Input: part model. Units: mm. Frame: model coordinates. Coordinates: 2 decimals unless noted, no trailing zeros. Write each loop counter-clockwise with the first axis right and the second up, starting at its lowest first coordinate (ties: lowest second). Pieces come first, ordered by that corner, then holes. Notation, with made-up numbers: M 71.5,28.25 L 95.5,28.25 A14 cw 95.5,55.25 Z; hole C 87,43.25 d8. An arc over 180 degrees is marked long. Use one line per item in the form item = value.
from build123d import *

# Parameters (mm, degrees)
SKETCH_1_W          = 207
SKETCH_1_H          = 75
EXTRUDE_1_DEPTH     = 1
SKETCH_2_R          = 3.3
CUT_EXTRUDE_1_DEPTH = 111.088600681
FILLET_1_R          = 5


with BuildPart() as part:
    # 草图1 → 凸台-拉伸1 (new body)
    with BuildSketch(Plane.XY):
        Rectangle(SKETCH_1_W, SKETCH_1_H)
    extrude(amount=EXTRUDE_1_DEPTH)

    # 草图2 → 切除-拉伸1 (cut, through all)
    with BuildSketch(Plane.XY.offset(1)):
        with Locations((-78.5, 29.5)):
            Circle(SKETCH_2_R)
        with Locations((78.5, 29.5)):
            Circle(SKETCH_2_R)
        with Locations((-78.5, -29.5)):
            Circle(SKETCH_2_R)
        with Locations((78.5, -29.5)):
            Circle(SKETCH_2_R)
    extrude(amount=-CUT_EXTRUDE_1_DEPTH, mode=Mode.SUBTRACT)

    # 圆角1
    fillet_1_edges = [part.edges().sort_by_distance(p)[0] for p in [
        (103.5, -37.5, 0.5),
        (-103.5, -37.5, 0.5),
        (-103.5, 37.5, 0.5),
        (103.5, 37.5, 0.5),
    ]]
    fillet(fillet_1_edges, radius=FILLET_1_R)


solid = part.part
(1) Pull-direction query (X, two-part tool) for faces 1 (the cylindrical face through (102, 36.07, 0.51)), 2 (the cylindrical face through (-81.8, 29.6, 0.5)), 3 (the flat face through (-1, 1, 1)); classes: pulls with the +X half, pulls with the -X half, needs draft (parallel to the pull), parting line crosses it, or undercut.
Computed:
face_1 = pulls with the +X half
face_2 = undercut
face_3 = needs draft
(2) Section query B-B on y = -29.5. Return the cut outline in (x, z).
Computed:
outline = M -103.5,0 L -81.8,0 L -81.8,1 L -103.5,1 Z; M -75.2,0 L 75.2,0 L 75.2,1 L -75.2,1 Z; M 81.8,0 L 103.5,0 L 103.5,1 L 81.8,1 Z
(3) Section query A-A on x = -78.5. Return the cut outline in (y, z), plus the area to 3 significant figures.
Computed:
outline = M -37.5,0 L -32.8,0 L -32.8,1 L -37.5,1 Z; M -26.2,0 L 26.2,0 L 26.2,1 L -26.2,1 Z; M 32.8,0 L 37.5,0 L 37.5,1 L 32.8,1 Z
area = 61.8 mm^2
(4) Line query: probe 1 along Y at (x, z) = (78.5, 0.45). Output: solid intervals per line, ascending.
Computed:
probe_1 = -37.5 to -32.8, -26.2 to 26.2, 32.8 to 37.5
